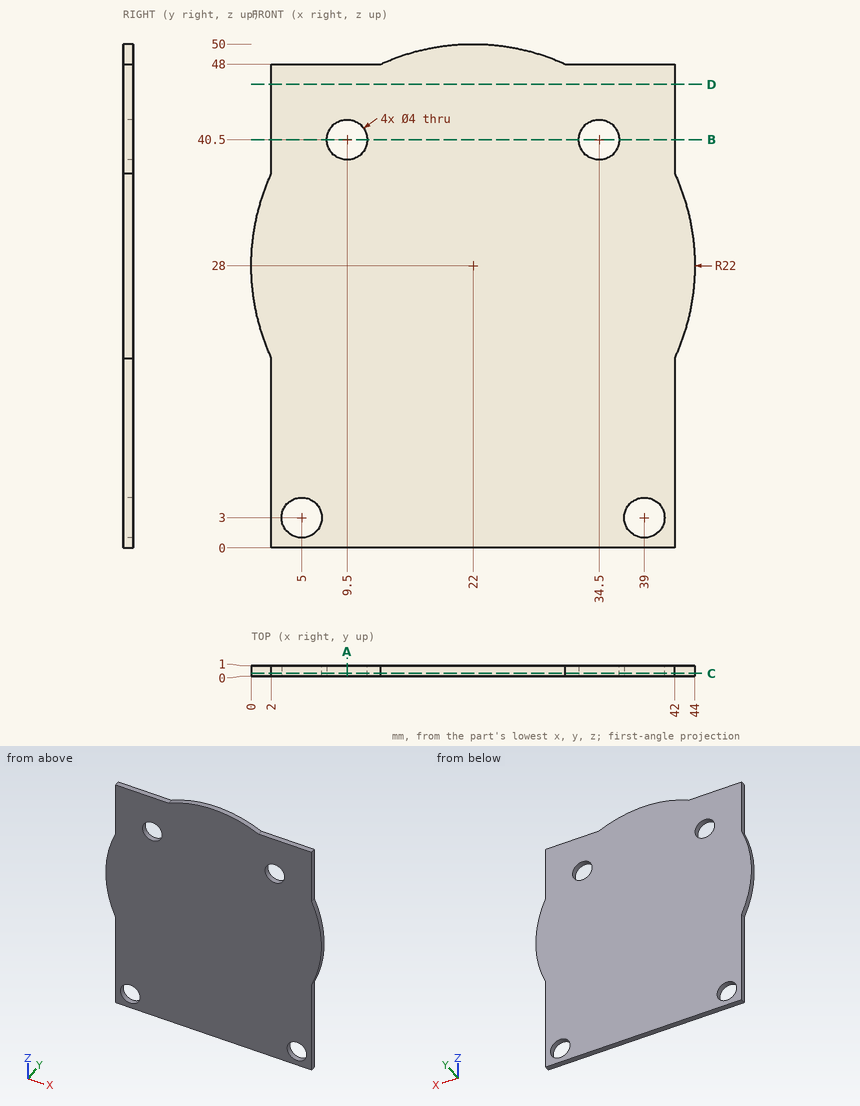
Print and shaded views of the part. All mm, measured from the part's lowest x, y and z. Give positions to 0.01 mm unless a question says otherwise; leave off trailing zeros. Loops run counter-clockwise (first coordinate to the right, second up) from the corner with the lowest first, then second, coordinate; pieces in that order, holes last. Notation, with made-up numbers: (-19, 89) - (16, 89) arc R29 ccw to (16, 128) - close; hole circle Ø10 at (-25.5, 49.25). An arc over 180 degrees is marked (long way). Use a Markdown table: item, result.
(1) Band-saw the part on D-D (z = 46). Give the cut face in (x, y), and give its area (3 significant figures).
Taken from the geometry:
| item | result |
|---|---|
| outline | (2, 0) - (42, 0) - (42, 1) - (2, 1) - close |
| area | 40.0 mm2 |
(2) Band-saw the part on B-B (z = 40.5). Give the cut face in (x, y).
Taken from the geometry:
| item | result |
|---|---|
| outline | (2, 0) - (7.5, 0) - (7.5, 1) - (2, 1) - close; (11.5, 0) - (32.5, 0) - (32.5, 1) - (11.5, 1) - close; (36.5, 0) - (42, 0) - (42, 1) - (36.5, 1) - close |
(3) Wall check: line 1 along X through (y, z) = (0.35, 40.5); line 2 along Z through (x, y) = (39, 0.8); line 3 along Z through (x, y) = (34.5, 0.3). Give the ranges that are in metal, low to high.
Taken from the geometry:
| item | result |
|---|---|
| line 1 | 2 to 7.5, 11.5 to 32.5, 36.5 to 42 |
| line 2 | 0 to 1, 5 to 48 |
| line 3 | 0 to 38.5, 42.5 to 48 |
(4) Band-saw the part on C-C (y = 0.25). Give the cut face in (x, z).
Taken from the geometry:
| item | result |
|---|---|
| outline | (2, 0) - (42, 0) - (42, 18.83) arc R22 ccw to (42, 37.17) - (42, 48) - (31.17, 48) arc R22 ccw to (12.83, 48) - (2, 48) - (2, 37.17) arc R22 ccw to (2, 18.83) - close; hole circle Ø4 at (5, 3); hole circle Ø4 at (9.5, 40.5); hole circle Ø4 at (34.5, 40.5); hole circle Ø4 at (39, 3) |
(5) Band-saw the part on A-A (x = 9.5). Give the cut face in (y, z), and give its area (3 significant figures).
Taken from the geometry:
| item | result |
|---|---|
| outline | (0, 0) - (1, 0) - (1, 38.5) - (0, 38.5) - close; (0, 42.5) - (1, 42.5) - (1, 48) - (0, 48) - close |
| area | 44.0 mm2 |
